Input: part model. Units: mm. Frame: model coordinates. A direction names the side the tool comes from. Coordinates: 2 decimals unless noted, no trailing zeros. Order: outer loops, then holes, each group sorted by start corner. A loop starts at its lowest first (then second) coordinate and runs counter-clockwise, first axis right, second up. Notation, with made-up numbers: (-1.5, 65.5) - (34.5, 65.5) arc R8 cw to (34.5, 73.5) - close; hole circle Ø6 at (12.5, 27.5). An arc over 180 degrees is marked (long way). One line per question, with ' | ' between items.
from build123d import *

# Parameters (mm, degrees)
F1_DEPTH  = 100
F2_W      = 100
F2_H      = 2
F3_DEPTH  = 25
F4_R      = 2.5
F5_DEPTH  = 5
F6_DEPTH  = 5
F7_W      = 3
F7_H      = 5
F8_DEPTH  = 2
F9_W      = 100
F9_H      = 1
F10_DEPTH = 3
F11_R     = 1
F12_DEPTH = 2
F13_W     = 41.0935450345
F13_H     = 3.0485875905
F14_DEPTH = 1
F15_DEPTH = 2


with BuildPart() as f1:
    # F0 (on Right) → F1 (new body)
    with BuildSketch(Plane.YZ):
        Polygon((0, 0), (-52.8542138636, 0), (-52.8542138636, -2), (2, -2), (2, 13.6397993192), (0, 13.6397993192), align=None)
    extrude(amount=F1_DEPTH)

    # F2 (on face) → F3 (join)
    with BuildSketch(Plane.XZ):
        with Locations((50, 12.6397993192)):
            Rectangle(F2_W, F2_H)
    extrude(amount=F3_DEPTH)

    # F4 (on face) → F5 (join)
    with BuildSketch(Plane.XY):
        with Locations((15, -42.8542138636)):
            Circle(F4_R)
    extrude(amount=F5_DEPTH)

    # F4 (on face) → F6 (join)
    with BuildSketch(Plane.XY):
        with Locations((15, -42.8542138636)):
            Circle(F4_R)
        with Locations((85, -42.8542138636)):
            Circle(F4_R)
        with Locations((15, -8)):
            Circle(F4_R)
        with Locations((85, -8)):
            Circle(F4_R)
    extrude(amount=F6_DEPTH)

    # F7 (on face) → F8 (cut, through all)
    with BuildSketch(Plane.XY.offset(13.6397993192)):
        with Locations((54.5849918723, -13.0749022961)):
            Rectangle(F7_W, F7_H)
        with Locations((44.6058220565, -13.0749022961)):
            Rectangle(F7_W, F7_H)
    extrude(amount=-F8_DEPTH, mode=Mode.SUBTRACT)

    # F9 (on face) → F10 (join)
    with BuildSketch(Plane.XZ.offset(25)):
        with Locations((50, 12.1397993192)):
            Rectangle(F9_W, F9_H)
    extrude(amount=F10_DEPTH)

    # F11 (on face) → F12 (cut, through all)
    with BuildSketch(Plane(origin=(0, 2, 0), x_dir=(-1, 0, 0), z_dir=(0, 1, 0))):
        with Locations((-69.4787353277, 8.7301367894)):
            Circle(F11_R)
        with Locations((-38.3921302855, 8.7301367894)):
            Circle(F11_R)
    extrude(amount=-F12_DEPTH, mode=Mode.SUBTRACT)

    # F13 (on face) → F14 (join)
    with BuildSketch(Plane.XY.offset(5)):
        Polygon((0.119697972, 0), (0.119697972, -52.5318421423), (27.1094348282, -52.5318421423), (27.1094348282, -49.4832545519), (68.2029798627, -49.4832545519), (68.2029798627, -52.5318421423), (100.119697972, -52.5318421423), (100.119697972, 0), align=None)
        with Locations((47.6562073454, -51.0075483471)):
            Rectangle(F13_W, F13_H)
    extrude(amount=F14_DEPTH)

    # F13 (on face) → F15 (join)
    with BuildSketch(Plane.XY.offset(5)):
        with Locations((47.6562073454, -51.0075483471)):
            Rectangle(F13_W, F13_H)
    extrude(amount=F15_DEPTH)


solid = f1.part
Item 1: Ray query, line 1 (Z direction, x = 9, y = -5); line 2 (Z direction, x = 50, y = -48); line 3 (Y direction, x = 14.5, z = 4). Return the intervals inside material, ascending.
Data:
line 1: -2 to 0, 5 to 6, 11.64 to 13.64 | line 2: -2 to 0, 5 to 6 | line 3: -45.3 to -40.4, -10.45 to -5.55, 0 to 2
Item 2: Section B-B on y = -32. Return the cut outline in (x, z), and give its area (3 significant figures).
Data:
outline: (0, -2) - (100, -2) - (100, 0) - (0, 0) - close; (0.12, 5) - (100.12, 5) - (100.12, 6) - (0.12, 6) - close | area: 300 mm^2
Item 3: Access query for faces 1 (the face through (47, -51, 7)), 2 (the face through (82.502, -42.744, 2.465)), 3 (the face through (49, -11, 13.64)), 4 (the face through (55, -10.575, 13)), 5 (the face through (49, -52.854, -1)). Directions: +Z, -Z, +X, -X, +Y, -Y. A direction counts if a zero-diameter tool reaches every point of the face in a straight line with its end or side. Return the directions, or none.
Data:
face 1: +Z, +X, -X, -Y | face 2: none | face 3: +Z, +X, -X, +Y, -Y | face 4: +Z | face 5: +Z, -Z, +X, -X, -Y
Item 4: Section D-D on y = -22. Return the cut outline in (x, z), and give its area (3 significant figures).
Data:
outline: (0, -2) - (100, -2) - (100, 0) - (0, 0) - close; (0, 11.64) - (100, 11.64) - (100, 13.64) - (0, 13.64) - close; (0.12, 5) - (100.12, 5) - (100.12, 6) - (0.12, 6) - close | area: 500 mm^2
Item 5: Section A-A on y = -8. Return the cut outline in (x, z).
Data:
outline: (0, -2) - (100, -2) - (100, 0) - (87.5, 0) - (87.5, 5) - (100.12, 5) - (100.12, 6) - (0.12, 6) - (0.12, 5) - (12.5, 5) - (12.5, 0) - (0, 0) - close; (0, 11.64) - (100, 11.64) - (100, 13.64) - (0, 13.64) - close; hole (17.5, 0) - (82.5, 0) - (82.5, 5) - (17.5, 5) - close
Item 6: Section C-C on x = 85. Return the cut outline in (y, z).
Data:
outline: (-52.85, -2) - (2, -2) - (2, 13.64) - (-25, 13.64) - (-25, 12.64) - (-28, 12.64) - (-28, 11.64) - (0, 11.64) - (0, 6) - (-52.53, 6) - (-52.53, 5) - (-45.35, 5) - (-45.35, 0) - (-52.85, 0) - close; hole (-40.35, 0) - (-10.5, 0) - (-10.5, 5) - (-40.35, 5) - close; hole (-5.5, 0) - (0, 0) - (0, 5) - (-5.5, 5) - close
Item 7: Contact query for flat-ended pins moving along their axis: P1, Ø1.5, axis at y = -4.5, z = 5.5, coming from the -X side; P2, Ø1, axis at y = -13, z = 12.5, coming from the -X side; P3, Ø3.5, axis at x = 73.5, z = 5, coming from the -Y side; P4, Ø0.8, axis at x = 68, z = 13, coming from the -Y side. Output: stop coordinate, or through.
Data:
P1: x = 0.12 | P2: x = 0 | P3: y = -52.53 | P4: y = -28
Item 8: Draft query along Z for faces 6 (the face through (83, -9.5, 2.5)), 7 (the face through (49, -26, -2)), 8 (the face through (56.085, -13, 13)). Return one class per face: released by +Z, released by -Z, zero draft, split by the parting line, or undercut.
Data:
face 6: undercut | face 7: released by -Z | face 8: zero draft
